```python
from build123d import *

# Parameters (mm, degrees)
ESQUISSE1_W                  = 10
ESQUISSE1_H                  = 10
ESQUISSE1_R                  = 4
ESQUISSE1_R_2                = 3
ESQUISSE1_W_2                = 1
BOSS_EXTRU_1_DEPTH           = 1
ESQUISSE2_R                  = 4
BOSS_EXTRU_2_DEPTH           = 10
CHANFREIN1_SIZE              = 1
ENL_V_MAT_EXTRU_1_REACH      = 15.491
ENL_V_MAT_EXTRU_1_END_RADIUS = 4
ESQUISSE3_W                  = 0.41236409
ESQUISSE3_H                  = 6.00446502
ESQUISSE3_H_2                = 0.99776749
R_P_TITION_CIRCULAIRE1_COUNT = 10
ESQUISSE9_W                  = 4
ESQUISSE9_H                  = 10
BOSS_EXTRU_8_DEPTH           = 1
CHANFREIN2_SIZE              = 1


with BuildPart() as part:
    # Esquisse1 → Boss.-Extru.1 (new body)
    # profile 1 of 5: a face of its own
    with BuildSketch(Plane.XY):
        Rectangle(ESQUISSE1_W, ESQUISSE1_H)
        Circle(ESQUISSE1_R, mode=Mode.SUBTRACT)
    # profile 2 of 5: a face of its own
    with BuildSketch(Plane.XY):
        Circle(ESQUISSE1_R)
        Circle(ESQUISSE1_R_2, mode=Mode.SUBTRACT)
    # profile 3 of 5: a face of its own
    with BuildSketch(Plane.XY):
        with BuildLine():
            Line((2.828427125, 1), (-2.828427125, 1))
            ThreePointArc((-2.828427125, 1), (-3, 0), (-2.828427125, -1))
            Line((-2.828427125, -1), (2.828427125, -1))
            ThreePointArc((2.828427125, -1), (2.956795679, -0.507305936), (3, 0))
            ThreePointArc((3, 0), (2.956795679, 0.507305936), (2.828427125, 1))
        make_face()
    # profile 4 of 5: a face of its own
    with BuildSketch(Plane.XY):
        with Locations((-5.5, 0)):
            Rectangle(ESQUISSE1_W_2, ESQUISSE1_H)
    # profile 5 of 5: a face of its own
    with BuildSketch(Plane.XY):
        with Locations((5.5, 0)):
            Rectangle(ESQUISSE1_W_2, ESQUISSE1_H)
    extrude(amount=BOSS_EXTRU_1_DEPTH)

    # Esquisse2 → Boss.-Extru.2 (add)
    with BuildSketch(Plane.XY.offset(1)):
        Circle(ESQUISSE2_R)
        with BuildLine():
            ThreePointArc((2.828427125, 1), (2.956795679, 0.507305936), (3, 0))
            ThreePointArc((3, 0), (2.956795679, -0.507305936), (2.828427125, -1))
            ThreePointArc((2.828427125, -1), (0, -3), (-2.828427125, -1))
            ThreePointArc((-2.828427125, -1), (-3, 0), (-2.828427125, 1))
            ThreePointArc((-2.828427125, 1), (0, 3), (2.828427125, 1))
        make_face(mode=Mode.SUBTRACT)
    extrude(amount=BOSS_EXTRU_2_DEPTH)

    # Chanfrein1
    chanfrein1_edges = [part.edges().sort_by_distance(p)[0] for p in [
        (-4, 0, 1),
    ]]
    chamfer(chanfrein1_edges, length=CHANFREIN1_SIZE - 0.0001)  # a hair under: the kernel refuses the full size

    # Enlèv. mat.-Extru.1: up to this cylinder (the profile starts inside it)
    enl_v_mat_extru_1_end = Plane(origin=(0, 0, 6.3335195), z_dir=(0, 0, -1)) * Cylinder(ENL_V_MAT_EXTRU_1_END_RADIUS, 46.651271, mode=Mode.PRIVATE)
    # Esquisse3 → Enlèv. mat.-Extru.1 (cut, up to the surface)
    with BuildSketch(Plane(origin=(0, 0, 0), x_dir=(1, 0, 0), z_dir=(0, 1, 0)), mode=Mode.PRIVATE) as enl_v_mat_extru_1_sk1:
        with Locations((0, -6.5)):
            Rectangle(ESQUISSE3_W, ESQUISSE3_H)
    enl_v_mat_extru_1_tool1 = extrude(enl_v_mat_extru_1_sk1.sketch, amount=ENL_V_MAT_EXTRU_1_REACH, mode=Mode.PRIVATE) & enl_v_mat_extru_1_end
    # Esquisse3 → Enlèv. mat.-Extru.1 (cut, up to the surface)
    with BuildSketch(Plane(origin=(0, 0, 0), x_dir=(1, 0, 0), z_dir=(0, 1, 0)), mode=Mode.PRIVATE) as enl_v_mat_extru_1_sk2:
        with Locations((0, -2.998883745)):
            Rectangle(ESQUISSE3_W, ESQUISSE3_H_2)
    enl_v_mat_extru_1_tool2 = extrude(enl_v_mat_extru_1_sk2.sketch, amount=ENL_V_MAT_EXTRU_1_REACH, mode=Mode.PRIVATE) & enl_v_mat_extru_1_end
    # Esquisse3 → Enlèv. mat.-Extru.1 (cut, up to the surface)
    with BuildSketch(Plane(origin=(0, 0, 0), x_dir=(1, 0, 0), z_dir=(0, 1, 0)), mode=Mode.PRIVATE) as enl_v_mat_extru_1_sk3:
        Polygon((-0.206182045, -9.50223251), (0.206182045, -9.50223251), (0, -10), align=None)
    enl_v_mat_extru_1_tool3 = extrude(enl_v_mat_extru_1_sk3.sketch, amount=ENL_V_MAT_EXTRU_1_REACH, mode=Mode.PRIVATE) & enl_v_mat_extru_1_end
    enl_v_mat_extru_1 = enl_v_mat_extru_1_tool1.solids().sort_by_distance((0, 0, 6.5))[0] + enl_v_mat_extru_1_tool2.solids().sort_by_distance((0, 0, 2.998884))[0] + enl_v_mat_extru_1_tool3.solids().sort_by_distance((0, 0, 9.668155))[0]
    add(enl_v_mat_extru_1, mode=Mode.SUBTRACT)

    # Répétition circulaire1: Enlèv. mat.-Extru.1 ×10 about axis
    r_p_tition_circulaire1_axis = Axis((0, 0, 0), (0, 0, 1))
    for i in range(1, R_P_TITION_CIRCULAIRE1_COUNT):
        add(enl_v_mat_extru_1.rotate(r_p_tition_circulaire1_axis, i * 360 / R_P_TITION_CIRCULAIRE1_COUNT), mode=Mode.SUBTRACT)

    # Esquisse9 → Boss.-Extru.8 (add)
    with BuildSketch(Plane(origin=(0, 0, 0), x_dir=(-1, 0, 0), z_dir=(0, 0, -1))):
        with Locations((-7, 0)):
            Rectangle(ESQUISSE9_W, ESQUISSE9_H)
        with Locations((7, 0)):
            Rectangle(ESQUISSE9_W, ESQUISSE9_H)
    extrude(amount=BOSS_EXTRU_8_DEPTH)

    # Chanfrein2
    chanfrein2_edges = [part.edges().sort_by_distance(p)[0] for p in [
        (6, 0, 0),
        (5, 0, -1),
        (-6, 0, 0),
        (-5, 0, -1),
        (-9, 0, 0),
        (9, 0, 0),
    ]]
    chamfer(chanfrein2_edges, length=CHANFREIN2_SIZE - 0.0001)  # a hair under: the kernel refuses the full size

    # Chanfrein3: read off the stored shape, not the designer's step
    # Chanfrein3 outline → Chanfrein3 (revolve, cut)
    with BuildSketch(Plane.XZ):
        Polygon((3, 11), (3, 10.5), (3.5, 11), align=None)
    revolve(axis=Axis((0, 0, 0), (0, 0, 1)), mode=Mode.SUBTRACT)


solid = part.part
```
The listing builds one solid part. Answer for the finished solid, in the listing's coordinates (mm). A direction names the side the tool comes from. Coordinates: 2 decimals unless noted, no trailing zeros. Loops run counter-clockwise (first coordinate to the right, second up) from the corner with the lowest first, then second, coordinate; pieces in that order, holes last. Notation, with made-up numbers: (-2.5, -23) - (14.5, -23) arc R28 ccw to (14.5, 7) - close; hole circle Ø7 at (88, 63). An arc over 180 degrees is marked (long way). Use a Markdown table: item, result. Add a question column.
1) The part is cut by section A-A, the plane z = 0.25. Give the vertices of the cut face in (x, y).
2) The mould has two halves that part along X. Classify faces 4 (the flat face through (-3.252, -1.274, 6.05)), 5 (the flat face through (-5.5, -0.1, -0.5)), 6 (the flat face through (0, 0, 0)), 7 (the flat face through (8, 0, -1)): released by +X, released by -X, zero draft, split by the parting line, or undercut.
3) Given pin 1 (3 mm diameter, centred on x = 1.5, z = 9, fed in from +Y); pin 2 (1.1 mm diameter, centred on y = -3.5, z = 5.5, fed in from -X); pin 3 (1 mm diameter, centred on x = -0.5, y = -0.5, fed in from +Z); pin 4 (3 mm diameter, centred on x = 6, z = 5.5, fed in from -Y), each flat-ended and moving along its own axis, determine where each tip first touches the part or whether it passes through.
4) The part is cut by section C-C, the plane x = -7.5. Give the vertices of the cut face in (y, z).
5) Find the intervals of material crossed by line 1 (Y direction, x = -3.5, z = 4.75); line 2 (Y direction, x = -2.25, z = 7); line 3 (Z direction, x = -7.75, y = -3.75), in increasing order.
6) The part is cut by section B-B, the plane z = 4.25. State how many separate pieces and enclosed holes the cut face has, and give its area (3 significant figures).
7) For faces 1 (the flat face through (-0.206, 3.5, 6.1)), 2 (the flat face through (-1.88, 2.94, 6.05)), 3 (the flat face through (0, -1, 0.5)), determine the directions among +Z, -Z, +X, -X, +Y, -Y from which every point of the face is accessible in a straight line to the end or side of a thin tool.
Here are the results:
| question | item | result |
|---|---|---|
| 1 | outline | (-6.75, -5) - (6.75, -5) - (6.75, 5) - (-6.75, 5) - close; hole (-2.83, -1) arc R3 ccw to (2.83, -1) - close; hole (-2.83, 1) - (2.83, 1) arc R3 ccw to start |
| 2 | face 4 | released by -X |
| 2 | face 5 | undercut |
| 2 | face 6 | undercut |
| 2 | face 7 | zero draft |
| 3 | pin 1 | stops at y = 4 |
| 3 | pin 2 | stops at x = -2.7 |
| 3 | pin 3 | stops at z = 1 |
| 3 | pin 4 | passes through |
| 4 | outline | (-5, -1) - (5, -1) - (5, 0) - (-5, 0) - close |
| 5 | line 1 | y = -1.94 to -1.35, -0.92 to 0.92, 1.35 to 1.94 |
| 5 | line 2 | y = -2.75 to -1.98, 1.98 to 2.75 |
| 5 | line 3 | z = -1 to 0 |
| 6 | separate pieces | 10 |
| 6 | enclosed holes | 0 |
| 6 | area | 17.9 mm^2 |
| 7 | face 1 | +Y, -Y |
| 7 | face 2 | none |
| 7 | face 3 | +Z, -Z |
